Work out the finished part from the listing and answer in its coordinate system (mm). Face numbers are marked on the shaded views. A direction names the side the tool comes from. Round coordinates to 2 decimals unless told otherwise and drop trailing zeros. Write each loop counter-clockwise with the first axis right and the second up, starting at its lowest first coordinate (ties: lowest second). Pieces come first, ordered by that corner, then holes.
1. Determine the mould class of the marked faces 1, 2 and 3 for opening direction Z: pulls with the +Z half, pulls with the -Z half, needs draft (parallel to the pull), parting line crosses it, or undercut.
2. Find section D-D (y = 28). Write down the section's boundary in (x, z), and give its area (3 significant figures).
3. Find section C-C (x = 17.5). Write down the section's boundary in (y, z), and give its area (3 significant figures).
4. Find section B-B (x = 26.5). Write down the section's boundary in (y, z).
5. Straight lines are drawn through the part: probe 1 along X at (y, z) = (1.1, -5); probe 2 along Y at (x, z) = (29.05, -35); probe 3 along Z at (x, y) = (27, 37). For each, find the intervals that lie inside material, in ascending order.
6. A tool of negligible diameter and unlimited length cuts with its end or side. For the marked faces 4 and 5, from which of +Z, -Z, +X, -X, +Y, -Y can it reach the whole face along a straight path? Write none if from no direction.
7. Find section A-A (y = 12.5). Write down the section's boundary in (x, z).
8. Flat-ended cylindrical pins translate along their axes: pin 1 Ø1.8 at (y, z) = (37.5, -5) entering from -X; pin 2 Ø12 at (x, z) = (10.5, -30) entering from +Y; pin 3 Ø10.5 at (y, z) = (21.5, -27) entering from -X. Find the tip coordinate at first contact, or state that the pin passes through.
```python
from build123d import *

# Parameters (mm, degrees)
SKETCH1_R           = 1.5
BOSS_EXTRUDE1_DEPTH = 5
SKETCH2_R           = 1.5
BOSS_EXTRUDE3_DEPTH = 5
FILLET4_R           = 3


with BuildPart() as part:
    # Sketch1 → Boss-Extrude1 (new body)
    with BuildSketch(Plane(origin=(0, 0, 0), x_dir=(1, 0, 0), z_dir=(0, 1, 0))):
        with BuildLine():
            Line((4.5, 0), (25, 0))
            Line((25, 0), (25, 40))
            Line((25, 40), (4.5, 40))
            ThreePointArc((4.5, 40), (1.318019485, 38.681980515), (0, 35.5))
            Line((0, 35.5), (0, 4.5))
            ThreePointArc((0, 4.5), (1.318019485, 1.318019485), (4.5, 0))
        make_face()
        with Locations(Location((7.5, 35, 0), (0, 0, 270))):
            Circle(SKETCH1_R, mode=Mode.SUBTRACT)
        with Locations(Location((17.5, 35, 0), (0, 0, 270))):
            Circle(SKETCH1_R, mode=Mode.SUBTRACT)
        with Locations(Location((17.5, 5, 0), (0, 0, 90))):
            Circle(SKETCH1_R, mode=Mode.SUBTRACT)
        with Locations(Location((7.5, 5, 0), (0, 0, 90))):
            Circle(SKETCH1_R, mode=Mode.SUBTRACT)
    extrude(amount=BOSS_EXTRUDE1_DEPTH)

    # Sketch2 → Boss-Extrude3 (add)
    with BuildSketch(Plane(origin=(25, 0, 0), x_dir=(0, 0, -1), z_dir=(1, 0, 0))):
        with BuildLine():
            Line((0, 0), (40, 0))
            Line((40, 0), (40, 38))
            ThreePointArc((40, 38), (38.681980515, 41.181980515), (35.5, 42.5))
            Line((35.5, 42.5), (4.5, 42.5))
            ThreePointArc((4.5, 42.5), (1.318019485, 41.181980515), (0, 38))
            Line((0, 38), (0, 0))
        make_face()
        with Locations((5, 37.5)):
            Circle(SKETCH2_R, mode=Mode.SUBTRACT)
        with Locations((5, 12.5)):
            Circle(SKETCH2_R, mode=Mode.SUBTRACT)
        with Locations(Location((35, 12.5, 0), (0, 0, 180))):
            Circle(SKETCH2_R, mode=Mode.SUBTRACT)
        with Locations(Location((35, 37.5, 0), (0, 0, 180))):
            Circle(SKETCH2_R, mode=Mode.SUBTRACT)
        with BuildLine():
            Line((27.5, 25), (12.5, 25))
            ThreePointArc((12.5, 25), (10.732233047, 24.267766953), (10, 22.5))
            Line((10, 22.5), (10, 5))
            Line((10, 5), (30, 5))
            Line((30, 5), (30, 22.5))
            ThreePointArc((30, 22.5), (29.267766953, 24.267766953), (27.5, 25))
        make_face(mode=Mode.SUBTRACT)
    extrude(amount=BOSS_EXTRUDE3_DEPTH)

    # Fillet4
    fillet4_edges = [part.edges().sort_by_distance(p)[0] for p in [
        (25, 5, -35),
        (25, 5, -5),
    ]]
    fillet(fillet4_edges, radius=FILLET4_R)


solid = part.part
```
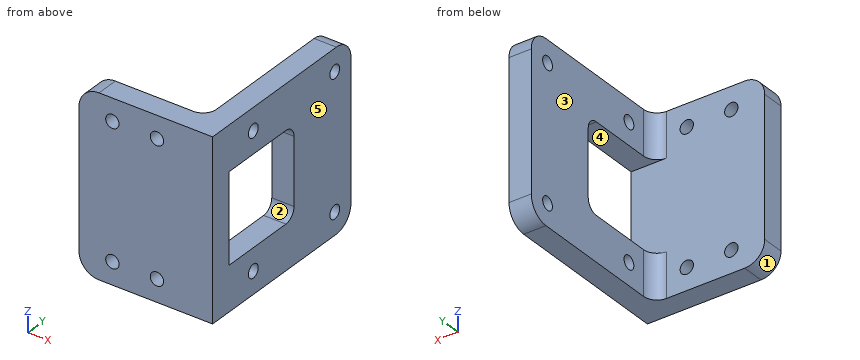
Worked answers:
1. face 1: pulls with the -Z half
1. face 2: undercut
1. face 3: needs draft
2. outline: (25, -40) - (30, -40) - (30, 0) - (25, 0) - close
2. area: 200 mm2
3. outline: (0, -40) - (5, -40) - (5, -36.5) - (0, -36.5) - close; (0, -33.5) - (5, -33.5) - (5, -6.5) - (0, -6.5) - close; (0, -3.5) - (5, -3.5) - (5, 0) - (0, 0) - close
3. area: 170 mm2
4. outline: (0, -40) - (38, -40) arc R4.5 ccw to (42.5, -35.5) - (42.5, -4.5) arc R4.5 ccw to (38, 0) - (0, 0) - close; hole (5, -30) - (22.5, -30) arc R2.5 ccw to (25, -27.5) - (25, -12.5) arc R2.5 ccw to (22.5, -10) - (5, -10) - close; hole circle Ø3 at (12.5, -35); hole circle Ø3 at (12.5, -5); hole circle Ø3 at (37.5, -35); hole circle Ø3 at (37.5, -5)
5. probe 1: x = 0 to 6, 9 to 16, 19 to 30
5. probe 2: y = 0 to 11, 14 to 36, 39 to 42.5
5. probe 3: z = -40 to -36.41, -33.59 to -6.41, -3.59 to 0
6. face 4: +X, -X
6. face 5: +Z, -Z, +X, +Y, -Y
7. outline: (25, -40) - (30, -40) - (30, -36.5) - (25, -36.5) - close; (25, -33.5) - (30, -33.5) - (30, -30) - (25, -30) - close; (25, -10) - (30, -10) - (30, -6.5) - (25, -6.5) - close; (25, -3.5) - (30, -3.5) - (30, 0) - (25, 0) - close
8. pin 1: passes through
8. pin 2: stops at y = 5
8. pin 3: stops at x = 25
